from build123d import *

# Parameters (mm, degrees)
SKETCH1_W           = 300
SKETCH1_H           = 180
BOSS_EXTRUDE1_DEPTH = 3
SKETCH2_W           = 40
SKETCH2_H           = 3
SKETCH2_W_2         = 3
SKETCH2_H_2         = 40
BOSS_EXTRUDE2_DEPTH = 3
SKETCH3_W           = 40
SKETCH3_H           = 3
CUT_EXTRUDE1_DEPTH  = 354.987287907
SKETCH4_W           = 40
SKETCH4_H           = 3
CUT_EXTRUDE2_DEPTH  = 3
SKETCH5_W           = 40
SKETCH5_H           = 3
CUT_EXTRUDE3_DEPTH  = 3
SKETCH6_W           = 40
SKETCH6_H           = 3
CUT_EXTRUDE4_DEPTH  = 3


with BuildPart() as part:
    # Sketch1 → Boss-Extrude1 (new body)
    with BuildSketch(Plane(origin=(0, 0, 0), x_dir=(0, 0, -1), z_dir=(1, 0, 0))):
        with Locations((-150, 90)):
            Rectangle(SKETCH1_W, SKETCH1_H)
    extrude(amount=BOSS_EXTRUDE1_DEPTH)

    # Sketch2 → Boss-Extrude2 (add)
    with BuildSketch(Plane(origin=(3, 0, 0), x_dir=(0, 0, -1), z_dir=(1, 0, 0))):
        with Locations((-270, 181.5)):
            Rectangle(SKETCH2_W, SKETCH2_H)
        with Locations((-30, 181.5)):
            Rectangle(SKETCH2_W, SKETCH2_H)
        with Locations((1.5, 150)):
            Rectangle(SKETCH2_W_2, SKETCH2_H_2)
        with Locations((1.5, 30)):
            Rectangle(SKETCH2_W_2, SKETCH2_H_2)
        with Locations((-30, -1.5)):
            Rectangle(SKETCH2_W, SKETCH2_H)
        with Locations((-270, -1.5)):
            Rectangle(SKETCH2_W, SKETCH2_H)
        with Locations((-301.5, 150)):
            Rectangle(SKETCH2_W_2, SKETCH2_H_2)
        with Locations((-301.5, 30)):
            Rectangle(SKETCH2_W_2, SKETCH2_H_2)
    extrude(amount=-BOSS_EXTRUDE2_DEPTH)

    # Sketch3 → Cut-Extrude1 (cut, through all)
    with BuildSketch(Plane(origin=(3, 0, 0), x_dir=(0, 0, -1), z_dir=(1, 0, 0))):
        with Locations((-246, 162.5)):
            Rectangle(SKETCH3_W, SKETCH3_H)
    extrude(amount=-CUT_EXTRUDE1_DEPTH, mode=Mode.SUBTRACT)

    # Sketch4 → Cut-Extrude2 (cut)
    with BuildSketch(Plane(origin=(3, 0, 0), x_dir=(0, 0, -1), z_dir=(1, 0, 0))):
        with Locations((-54, 162.5)):
            Rectangle(SKETCH4_W, SKETCH4_H)
    extrude(amount=-CUT_EXTRUDE2_DEPTH, mode=Mode.SUBTRACT)

    # Sketch5 → Cut-Extrude3 (cut)
    with BuildSketch(Plane(origin=(3, 0, 0), x_dir=(0, 0, -1), z_dir=(1, 0, 0))):
        with Locations((-246, 17.5)):
            Rectangle(SKETCH5_W, SKETCH5_H)
    extrude(amount=-CUT_EXTRUDE3_DEPTH, mode=Mode.SUBTRACT)

    # Sketch6 → Cut-Extrude4 (cut)
    with BuildSketch(Plane(origin=(3, 0, 0), x_dir=(0, 0, -1), z_dir=(1, 0, 0))):
        with Locations((-54, 17.5)):
            Rectangle(SKETCH6_W, SKETCH6_H)
    extrude(amount=-CUT_EXTRUDE4_DEPTH, mode=Mode.SUBTRACT)


solid = part.part
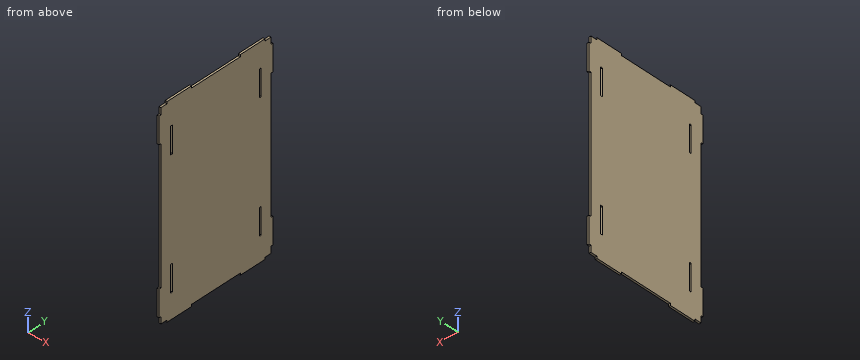
Geometry: final body of the model. Coordinates: model frame, mm. Coordinates: 2 decimals unless noted, no trailing zeros. Loops run counter-clockwise (first coordinate to the right, second up) from the corner with the lowest first, then second, coordinate; pieces in that order, holes last. Notation, with made-up numbers: (21, -35.75) - (54, -35.75) arc R12 ccw to (54, -18.75) - close; hole circle Ø6 at (-16, -8). An arc over 180 degrees is marked (long way). Put each result on its own line as item: value. Start each with the question number.
Q1. Cut plane B-B, the plane y = 116. Return loops of the section in (x, z).
Q2. Line query: line 1 (Y direction, x = 1.9, z = 54); line 2 (Y direction, x = 0.4, z = 45.5); line 3 (Y direction, x = 2.5, z = 128). Output: solid intervals per line, ascending.
Q3. Cut plane A-A, the plane z = 239.5. Return loops of the section in (x, y), and give its area (3 significant figures).
Q4. Cut plane C-C, the plane x = 2.4. Give the number of separate pieces and of enclosed holes in the cut face, and give its area (3 significant figures).
Q5. Cut plane D-D, the plane z = 137.5. Return loops of the section in (x, y).
Q6. Pin query (flat end, axial travel): pin 1 Ø0.9 at (x, y) = (1, 100) entering from +Z; pin 2 Ø0.9 at (x, y) = (1.5, 182) entering from -Z; pin 3 Ø1.5 at (x, y) = (1.5, 87.5) entering from -Z. Return the tip coordinate at first contact, or that it passes through.
Filled sheet:
1. outline: (0, 0) - (3, 0) - (3, 300) - (0, 300) - close
2. line 1: 0 to 16, 19 to 161, 164 to 180
2. line 2: -3 to 16, 19 to 161, 164 to 183
2. line 3: 0 to 180
3. outline: (0, 0) - (3, 0) - (3, 16) - (0, 16) - close; (0, 19) - (3, 19) - (3, 161) - (0, 161) - close; (0, 164) - (3, 164) - (3, 180) - (0, 180) - close
3. area: 522 mm²
4. separate pieces: 1
4. enclosed holes: 4
4. area: 54,500 mm²
5. outline: (0, 0) - (3, 0) - (3, 180) - (0, 180) - close
6. pin 1: z = 300
6. pin 2: z = 10
6. pin 3: z = 0
